Source: CAD feature listing. Evaluate the final solid. Frame: model axes, mm. Face numbers are marked on the shaded views. A direction names the side the tool comes from. Round coordinates to 2 decimals unless told otherwise and drop trailing zeros. Order: outer loops, then holes, each group sorted by start corner. A loop starts at its lowest first (then second) coordinate and runs counter-clockwise, first axis right, second up. Notation, with made-up numbers: (60, 69) - (95, 69) arc R4 ccw to (95, 73) - close; hole circle Ø4 at (45, 23.5). An arc over 180 degrees is marked (long way). Return JSON: item names as keys, results as strings. Group by question number.
1) Section B-B, the plane z = -2.25. Return loops of the section in (x, y), plus the area to 3 significant figures.
2) Ray query, line 1 (Y direction, x = 35, z = 7.5); line 2 (Z direction, x = -10.5, y = 1); line 3 (X direction, y = 7.75, z = 1.5). Return the intervals inside material, ascending. Write a range as from..to.
3) Access query for the marked faces 4, 5 and 6. Directions: +Z, -Z, +X, -X, +Y, -Y. A direction counts if a zero-diameter tool reaches every point of the face in a straight line with its end or side. Return the directions, or none.
4) Contact query for a flat-ended pin moving along its axis: P1, Ø7, axis at x = 35, y = 6, coming from the -Z side. Output: stop coordinate, or through.
5) Section A-A, the plane x = 35. Return loops of the section in (y, z).
6) Mould query, pull axis Z, two halves, no side actions, for the marked faces 1, 2 and 3. Classes: pulls with the +Z half, pulls with the -Z half, needs draft (parallel to the pull), parting line crosses it, or undercut.
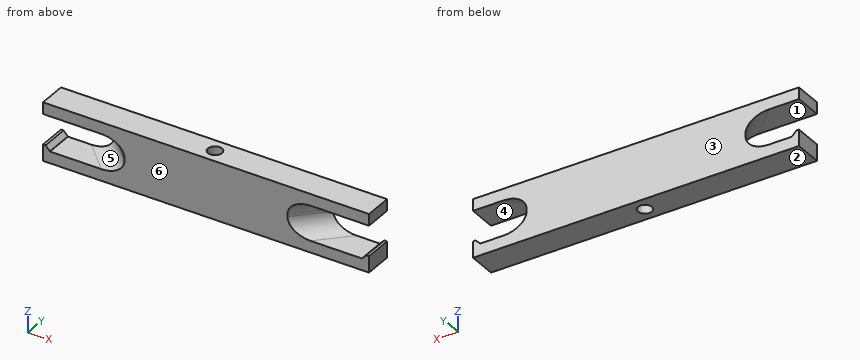
```python
from build123d import *

# Parameters (mm, degrees)
PAD_DEPTH    = 15
SKETCH001_W  = 140
SKETCH001_H  = 12
PAD001_DEPTH = 5
SKETCH002_W  = 140
SKETCH002_H  = 12
PAD002_DEPTH = 5
FILLET_R     = 7
SKETCH003_R  = 3
POCKET_DEPTH = 25.001
SKETCH004_W  = 3
SKETCH004_H  = 12
PAD003_DEPTH = 2
CHAMFER_SIZE = 1.9


with BuildPart() as part:
    # Sketch → Pad (new body)
    with BuildSketch(Plane.XY):
        Polygon((0, 0), (70, 0), (82, 12), (-12, 12), align=None)
    extrude(amount=PAD_DEPTH)

    # Sketch001 (on Face6 of Pad) → Pad001 (join)
    with BuildSketch(Plane.XY.offset(15)):
        with Locations((35, 6)):
            Rectangle(SKETCH001_W, SKETCH001_H)
    extrude(amount=PAD001_DEPTH)

    # Sketch002 (on Face11 of Pad001) → Pad002 (join)
    with BuildSketch(Plane(origin=(0, 0, 0), x_dir=(1, 0, 0), z_dir=(0, 0, -1))):
        with Locations((35, -6)):
            Rectangle(SKETCH002_W, SKETCH002_H)
    extrude(amount=PAD002_DEPTH)

    # Fillet
    fillet_edges = [part.edges().sort_by_distance(p)[0] for p in [
        (76, 6, 15),
        (-6, 6, 15),
        (-6, 6, 0),
        (76, 6, 0),
    ]]
    fillet(fillet_edges, radius=FILLET_R)

    # Sketch003 (on Face20 of Fillet) → Pocket (cut, through all)
    with BuildSketch(Plane.XY.offset(20)):
        with Locations((35, 6)):
            Circle(SKETCH003_R)
    extrude(amount=-POCKET_DEPTH, mode=Mode.SUBTRACT)

    # Sketch004 (on Face7 of Pocket) → Pad003 (join)
    with BuildSketch(Plane.XY):
        with Locations((-33.5, 6)):
            Rectangle(SKETCH004_W, SKETCH004_H)
        with Locations((103.5, 6)):
            Rectangle(SKETCH004_W, SKETCH004_H)
    extrude(amount=PAD003_DEPTH)

    # Chamfer
    chamfer_edges = [part.edges().sort_by_distance(p)[0] for p in [
        (-32, 6, 2),
        (102, 6, 2),
    ]]
    chamfer(chamfer_edges, length=CHAMFER_SIZE)


solid = part.part
```
Geometry check:
{
 "1": {"outline": "(-35, 0) - (105, 0) - (105, 12) - (-35, 12) - close; hole circle Ø6 at (35, 6)", "area": "1,650 mm2"},
 "2": {"line 1": "0..3, 9..12", "line 2": "-5..0.01, 14.99..20", "line 3": "-35..-33.4, -11.53..32.56, 37.44..81.53, 103.4..105"},
 "3": {"face 4": "+X, -Y", "face 5": "-Y", "face 6": "+Z, -Z, +X, -X, -Y"},
 "4": {"P1": "z = -5"},
 "5": {"outline": "(0, -5) - (3, -5) - (3, 20) - (0, 20) - close; (9, -5) - (12, -5) - (12, 20) - (9, 20) - close"},
 "6": {"face 1": "undercut", "face 2": "pulls with the -Z half", "face 3": "needs draft"}
}
